Geometry: final body of the model. Coordinates: model frame, mm. A direction names the side the tool comes from. Give positions to 0.01 mm unless a question says otherwise; leave off trailing zeros. Write each loop counter-clockwise with the first axis right and the second up, starting at its lowest first coordinate (ties: lowest second). Pieces come first, ordered by that corner, then holes.
Q1. Reachability of faces 4 (the flat face through (-26.08, -23.53, -1.97)), 5 (the flat face through (25.346, -25.099, -1.972)), 6 (the cylindrical face through (38.717, 21.875, -1.972)) from +Z, -Z, +X, -X, +Y, -Y: full face, straight path, thin tool, end or side. Return the list, or none.
Q2. Mould query, pull axis Y, two halves, no side actions, for faces 1 (the cylindrical face through (27.1, 31.93, -1.97)), 2 (the cylindrical face through (-14.541, -39.273, -1.972)), 3 (the flat face through (30.67, -1.36, -1.97)). Classes: +Y half, -Y half, draft (parallel to the pull), parting line (faces both ways), or undercut.
Q3. Pin query (flat end, axial travel): pin 1 Ø1 at (y, z) = (-16.5, -3.5) entering from -X; pin 2 Ø1 at (y, z) = (38.5, -2.5) entering from +X; pin 3 Ø2 at (x, z) = (-32, -2.5) entering from +Y. Return the tip coordinate at first contact, or that it passes through.
Q4. Section B-B (z = -1.65). State how many separate pieces and enclosed holes the cut face has, plus the area to 3 significant figures.
Q5. Line query: line 1 (X direction, y = 18, z = -1.7); line 2 (Y direction, x = 7.5, z = -2.2); line 3 (Y direction, x = -39, z = -2.4). Output: solid intervals per line, ascending.
Q6. Section A-A (y = 16). Return the cut outline in (x, z).
from build123d import *

# Parameters (mm, degrees)
SKETCH1_R          = 14
SKETCH1_R_2        = 1.75
SKETCH1_R_3        = 1.5
BASE_FLANGE1_DEPTH = 4


# Sheet-metal steps are written as plain solids
with BuildPart() as part:
    # Sketch1 → Base-Flange1 (new body)
    with BuildSketch(Plane.XY):
        with BuildLine():
            Line((-12.445814591, 28.677522558), (-2.085412981, 40.183914245))
            ThreePointArc((-2.085412981, 40.183914245), (0.269444296, 41.894818203), (3.116600797, 42.5))
            Line((3.116600797, 42.5), (13.5, 42.5))
            ThreePointArc((13.5, 42.5), (15.621320344, 41.621320344), (16.5, 39.5))
            Line((16.5, 39.5), (16.5, 37.5))
            ThreePointArc((16.5, 37.5), (15.621320344, 35.378679656), (13.5, 34.5))
            Line((13.5, 34.5), (4.5, 34.5))
            ThreePointArc((4.5, 34.5), (2.234136105, 32.234136105), (4.5, 29.96827221))
            Line((4.5, 29.96827221), (8.899509069, 29.96827221))
            Line((8.899509069, 29.96827221), (24.232203159, 32.123141835))
            ThreePointArc((24.232203159, 32.123141835), (27.135876357, 31.920097226), (29.705928134, 30.553576456))
            Line((29.705928134, 30.553576456), (37.660073394, 23.879256102))
            ThreePointArc((37.660073394, 23.879256102), (38.720294659, 21.842590001), (38.029843894, 19.652759943))
            Line((38.029843894, 19.652759943), (36.744268675, 18.120671057))
            ThreePointArc((36.744268675, 18.120671057), (34.707602574, 17.060449792), (32.517772516, 17.750900557))
            Line((32.517772516, 17.750900557), (25.623372528, 23.535989044))
            ThreePointArc((25.623372528, 23.535989044), (22.431150845, 23.256705835), (22.710434054, 20.064484152))
            Line((22.710434054, 20.064484152), (26.080653529, 17.236534234))
            Line((26.080653529, 17.236534234), (39.211302131, 9.031594352))
            ThreePointArc((39.211302131, 9.031594352), (41.305130289, 7.009608003), (42.395521552, 4.310794923))
            Line((42.395521552, 4.310794923), (44.198579902, -5.914857115))
            ThreePointArc((44.198579902, -5.914857115), (43.701612775, -8.156530957), (41.765101175, -9.390224907))
            Line((41.765101175, -9.390224907), (39.795485669, -9.737521262))
            ThreePointArc((39.795485669, -9.737521262), (37.553811827, -9.240554136), (36.320117877, -7.304042536))
            Line((36.320117877, -7.304042536), (34.757284278, 1.559227241))
            ThreePointArc((34.757284278, 1.559227241), (32.132380811, 3.397204436), (30.294403616, 0.772300968))
            Line((30.294403616, 0.772300968), (31.058370348, -3.560369672))
            Line((31.058370348, -3.560369672), (35.84299705, -18.285936503))
            ThreePointArc((35.84299705, -18.285936503), (36.147254703, -21.180754707), (35.247779262, -23.949055464))
            Line((35.247779262, -23.949055464), (30.056079661, -32.941342951))
            ThreePointArc((30.056079661, -32.941342951), (28.234460585, -34.33912043), (25.958003449, -34.039419162))
            Line((25.958003449, -34.039419162), (24.225952642, -33.039419162))
            ThreePointArc((24.225952642, -33.039419162), (22.828175163, -31.217800086), (23.127876431, -28.941342951))
            Line((23.127876431, -28.941342951), (27.627876431, -21.147114317))
            ThreePointArc((27.627876431, -21.147114317), (26.798512683, -18.051886675), (23.703285041, -18.881250422))
            Line((23.703285041, -18.881250422), (21.503530506, -22.69133704))
            Line((21.503530506, -22.69133704), (15.703355299, -37.047274443))
            ThreePointArc((15.703355299, -37.047274443), (14.07567691, -39.460406892), (11.60720932, -41.002876635))
            Line((11.60720932, -41.002876635), (1.850005711, -44.554208318))
            ThreePointArc((1.850005711, -44.554208318), (-0.443909504, -44.454053817), (-1.995132582, -42.761190886))
            Line((-1.995132582, -42.761190886), (-2.679172868, -40.881805644))
            ThreePointArc((-2.679172868, -40.881805644), (-2.579018367, -38.587890429), (-0.886155436, -37.036667352))
            Line((-0.886155436, -37.036667352), (7.571078151, -33.958486062))
            ThreePointArc((7.571078151, -33.958486062), (8.925322639, -31.054299386), (6.021135963, -29.700054898))
            Line((6.021135963, -29.700054898), (1.886949755, -31.20477562))
            Line((1.886949755, -31.20477562), (-11.78406092, -38.473780937))
            ThreePointArc((-11.78406092, -38.473780937), (-14.582066543, -39.276096138), (-17.464502862, -38.870996132))
            Line((-17.464502862, -38.870996132), (-27.221706472, -35.319664448))
            ThreePointArc((-27.221706472, -35.319664448), (-28.914569403, -33.768441371), (-29.014723904, -31.474526156))
            Line((-29.014723904, -31.474526156), (-28.330683618, -29.595140915))
            ThreePointArc((-28.330683618, -29.595140915), (-26.779460541, -27.902277983), (-24.485545325, -27.802123482))
            Line((-24.485545325, -27.802123482), (-16.028311738, -30.880304772))
            ThreePointArc((-16.028311738, -30.880304772), (-13.124125062, -29.526060284), (-14.47836955, -26.621873608))
            Line((-14.47836955, -26.621873608), (-18.612555757, -25.117152886))
            Line((-18.612555757, -25.117152886), (-33.757584069, -21.897977741))
            ThreePointArc((-33.757584069, -21.897977741), (-36.416698999, -20.714063497), (-38.364380059, -18.550944536))
            Line((-38.364380059, -18.550944536), (-43.556079661, -9.558657049))
            ThreePointArc((-43.556079661, -9.558657049), (-43.855780928, -7.282199914), (-42.458003449, -5.460580838))
            Line((-42.458003449, -5.460580838), (-40.725952642, -4.460580838))
            ThreePointArc((-40.725952642, -4.460580838), (-38.449495507, -4.16087957), (-36.627876431, -5.558657049))
            Line((-36.627876431, -5.558657049), (-32.127876431, -13.352885683))
            ThreePointArc((-32.127876431, -13.352885683), (-29.032648788, -14.18224943), (-28.203285041, -11.087021788))
            Line((-28.203285041, -11.087021788), (-30.403039576, -7.27693517))
            Line((-30.403039576, -7.27693517), (-39.935558458, 4.924132608))
            ThreePointArc((-39.935558458, 4.924132608), (-41.211553267, 7.540309666), (-41.313137454, 10.449300179))
            Line((-41.313137454, 10.449300179), (-39.510079105, 20.674952217))
            ThreePointArc((-39.510079105, 20.674952217), (-38.276385155, 22.611463816), (-36.034711312, 23.108430943))
            Line((-36.034711312, 23.108430943), (-34.065095806, 22.761134587))
            ThreePointArc((-34.065095806, 22.761134587), (-32.128584207, 21.527440637), (-31.63161708, 19.285766795))
            Line((-31.63161708, 19.285766795), (-33.194450679, 10.422497018))
            ThreePointArc((-33.194450679, 10.422497018), (-31.356473484, 7.797593551), (-28.731570017, 9.635570746))
            Line((-28.731570017, 9.635570746), (-27.967603284, 13.968241386))
            Line((-27.967603284, 13.968241386), (-27.427241211, 29.442186584))
            ThreePointArc((-27.427241211, 29.442186584), (-26.723063746, 32.266488135), (-24.93101869, 34.560201209))
            Line((-24.93101869, 34.560201209), (-16.97687343, 41.234521563))
            ThreePointArc((-16.97687343, 41.234521563), (-14.787043372, 41.924972328), (-12.750377271, 40.864751063))
            Line((-12.750377271, 40.864751063), (-11.464802052, 39.332662177))
            ThreePointArc((-11.464802052, 39.332662177), (-10.774351287, 37.142832119), (-11.834572552, 35.106166018))
            Line((-11.834572552, 35.106166018), (-18.72897254, 29.321077531))
            ThreePointArc((-18.72897254, 29.321077531), (-19.008255749, 26.128855848), (-15.816034066, 25.84957264))
            Line((-15.816034066, 25.84957264), (-12.445814591, 28.677522558))
        make_face()
        Circle(SKETCH1_R, mode=Mode.SUBTRACT)
        with Locations((0, 21.45)):
            Circle(SKETCH1_R_2, mode=Mode.SUBTRACT)
        with Locations((21.45, 0)):
            Circle(SKETCH1_R_2, mode=Mode.SUBTRACT)
        with Locations((0, -21.45)):
            Circle(SKETCH1_R_2, mode=Mode.SUBTRACT)
        with Locations((-21.45, 0)):
            Circle(SKETCH1_R_2, mode=Mode.SUBTRACT)
        with Locations((13.5, 38.5)):
            Circle(SKETCH1_R_3, mode=Mode.SUBTRACT)
        with Locations((35.088922955, 20.815078329)):
            Circle(SKETCH1_R_3, mode=Mode.SUBTRACT)
        with Locations((40.259348889, -6.609449825)):
            Circle(SKETCH1_R_3, mode=Mode.SUBTRACT)
        with Locations((26.591978046, -30.941342951)):
            Circle(SKETCH1_R_3, mode=Mode.SUBTRACT)
        with Locations((0.481925137, -40.795437835)):
            Circle(SKETCH1_R_3, mode=Mode.SUBTRACT)
        with Locations((-25.853625899, -31.560893965)):
            Circle(SKETCH1_R_3, mode=Mode.SUBTRACT)
        with Locations((-40.091978046, -7.558657049)):
            Circle(SKETCH1_R_3, mode=Mode.SUBTRACT)
        with Locations((-35.570848092, 19.980359506)):
            Circle(SKETCH1_R_3, mode=Mode.SUBTRACT)
        with Locations((-14.405722991, 38.170343791)):
            Circle(SKETCH1_R_3, mode=Mode.SUBTRACT)
    extrude(amount=-BASE_FLANGE1_DEPTH)


solid = part.part
Computed:
1. face 4: +Z, -Z, -X
1. face 5: +Z, -Z
1. face 6: +Z, -Z, +X
2. face 1: +Y half
2. face 2: -Y half
2. face 3: undercut
3. pin 1: stops at x = -39.84
3. pin 2: stops at x = 16.5
3. pin 3: stops at y = 22.35
4. separate pieces: 1
4. enclosed holes: 14
4. area: 4,120 mm2
5. line 1: x = -39.98 to -31.86, -27.83 to 25.17, 32.22 to 36.64
5. line 2: y = -42.5 to -33.98, -29.68 to -11.82, 11.82 to 29.97, 34.5 to 42.5
5. line 3: y = -17.45 to -8.59, -6.53 to -4.07, 3.73 to 21.89
6. outline: (-40.33, -4) - (-32.21, -4) - (-32.21, 0) - (-40.33, 0) - close; (-27.9, -4) - (28.06, -4) - (28.06, 0) - (-27.9, 0) - close
